Can you work these out from the drawing? Everything is in mm from the part's minimum corner. A direction names the side the tool comes from. Give positions to 0.01 mm unless a question says otherwise; leave off trailing zeros. Loops run counter-clockwise (first coordinate to the right, second up) from the corner with the lowest first, then second, coordinate; pieces in that order, holes last. Notation, with made-up numbers: (69.25, -29) -> (79.25, -29) arc R18 ccw to (79.25, -9) -> close; hole circle Ø4 at (-23.5, -4.5). An arc over 180 degrees is marked (long way). Write item = value, one per line. Start each with the question number.
1) I want a section at A-A (z = 117.5). List the corners of the cut face in (x, y) for me.
2) I need wall thicknesses on probe 1 along Y at (x, z) = (107, 122); probe 2 along X at (y, z) = (44, 108); probe 3 along Y at (x, z) = (184, 55). Which ranges of each line are inside material? Lowest first, please. Write a range as from..to.
3) On a 3-axis mill with a long thin cutter (end or side, diameter ignored), from which of +Z, -Z, +X, -X, +Y, -Y can I reach the whole of each face in a straight line? I mean the marked faces 4 and 5. Say none if no direction works.
4) I want a section at D-D (x = 184.15). List the corners of the cut face in (y, z) for me, and give its area (3 significant figures).
5) I want a section at C-C (y = 139.7). List the corners of the cut face in (x, z) for me.
6) I want a section at B-B (y = 44.45). List the corners of the cut face in (x, z) for me.
7) I'm going to push flat-ended pins straight in: pin 1 Ø6 at (x, z) = (28, 78) entering from +Y; pin 2 Ø8 at (x, y) = (134, 154.5) entering from -Z. Where does each tip first touch, or does it pass through?
8) If we mould it in two halves opening along Y, with no side actions, what happens to the marked faces 1, 2 and 3? For each: +Y half, -Y half, draft (parallel to the pull), parting line (faces both ways), or undercut.
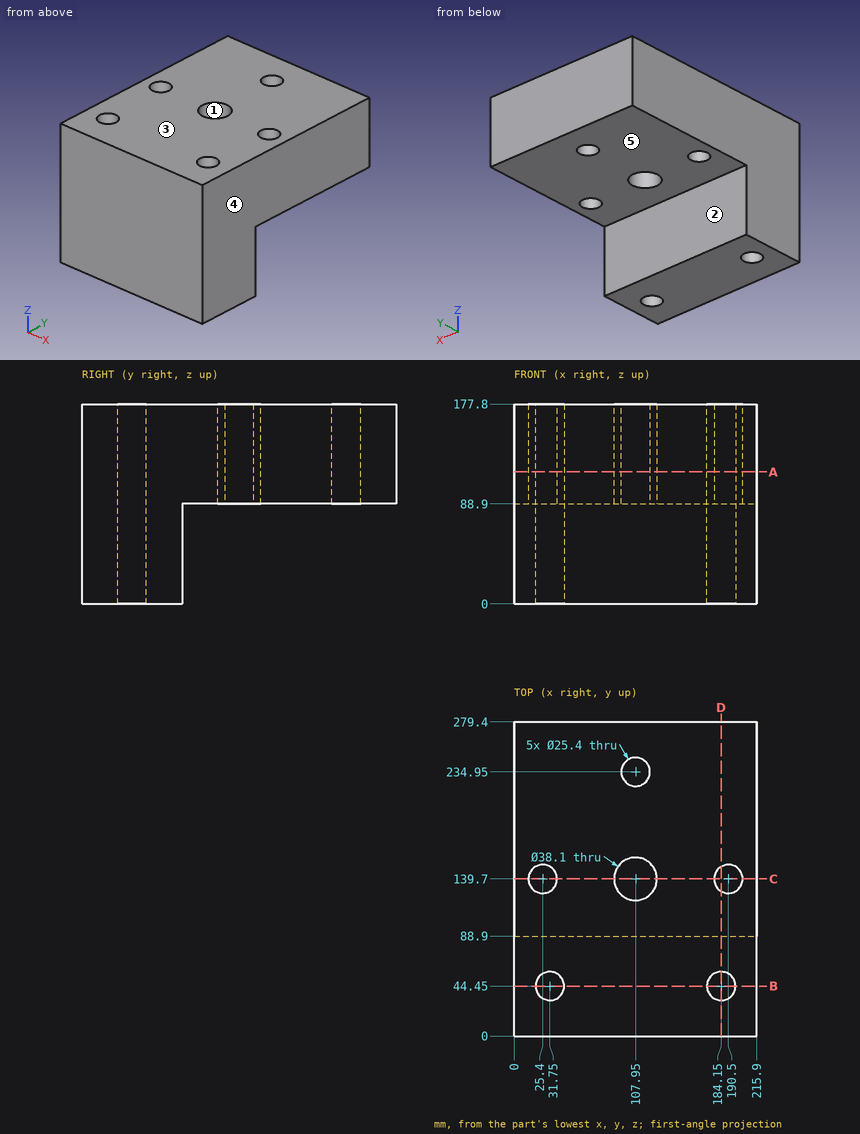
Answer list:
q1.outline = (0, 0) -> (215.9, 0) -> (215.9, 279.4) -> (0, 279.4) -> close; hole circle Ø25.4 at (25.4, 139.7); hole circle Ø25.4 at (31.75, 44.45); hole circle Ø38.1 at (107.95, 139.7); hole circle Ø25.4 at (107.95, 234.95); hole circle Ø25.4 at (184.15, 44.45); hole circle Ø25.4 at (190.5, 139.7)
q2.probe_1 = 0..120.67, 158.73..222.29, 247.61..279.4
q2.probe_2 = 0..19.06, 44.44..171.46, 196.84..215.9
q2.probe_3 = 0..31.75, 57.15..88.9
q3.face_4 = +Z, -Z, +X, +Y, -Y
q3.face_5 = -Z, +X, -X, +Y
q4.outline = (0, 0) -> (31.75, 0) -> (31.75, 177.8) -> (0, 177.8) -> close; (57.15, 0) -> (88.9, 0) -> (88.9, 88.9) -> (128.7, 88.9) -> (128.7, 177.8) -> (57.15, 177.8) -> close; (150.7, 88.9) -> (279.4, 88.9) -> (279.4, 177.8) -> (150.7, 177.8) -> close
q4.area = 26,300 mm^2
q5.outline = (0, 88.9) -> (12.7, 88.9) -> (12.7, 177.8) -> (0, 177.8) -> close; (38.1, 88.9) -> (88.9, 88.9) -> (88.9, 177.8) -> (38.1, 177.8) -> close; (127, 88.9) -> (177.8, 88.9) -> (177.8, 177.8) -> (127, 177.8) -> close; (203.2, 88.9) -> (215.9, 88.9) -> (215.9, 177.8) -> (203.2, 177.8) -> close
q6.outline = (0, 0) -> (19.05, 0) -> (19.05, 177.8) -> (0, 177.8) -> close; (44.45, 0) -> (171.45, 0) -> (171.45, 177.8) -> (44.45, 177.8) -> close; (196.85, 0) -> (215.9, 0) -> (215.9, 177.8) -> (196.85, 177.8) -> close
q7.pin_1 = 88.9
q7.pin_2 = 88.9
q8.face_1 = undercut
q8.face_2 = +Y half
q8.face_3 = draft
